from build123d import *
from build123d.topology import SkipClean

# Parameters (mm, degrees)
SZKIC1_W                   = 3.2
SZKIC1_H                   = 4.5
OBR_T1_ANGLE               = 180
OBR_T1_OTHER_WAY_ANGLE     = 180
WYTNIJ_WYCI_GNI_CIE1_DEPTH = 32.6


with BuildPart() as part:
    # Szkic1 → Obrót1 (revolve)
    with BuildSketch(Plane(origin=(0, 0, 0), x_dir=(1, 0, 0), z_dir=(0, 1, 0))):
        with Locations((1.6, 10.4)):
            Rectangle(SZKIC1_W, SZKIC1_H)
    revolve(axis=Axis((1, 0, 0), (-1, 0, 0)), revolution_arc=OBR_T1_ANGLE)

    # Szkic1 → Obrót1 other way (revolve)
    with SkipClean():  # the faces are left unmerged after this step: merging them gives an invalid solid
        with BuildSketch(Plane(origin=(0, 0, 0), x_dir=(1, 0, 0), z_dir=(0, 1, 0))):
            with Locations((1.6, 10.4)):
                Rectangle(SZKIC1_W, SZKIC1_H)
        revolve(axis=Axis((1, 0, 0), (1, 0, 0)), revolution_arc=OBR_T1_OTHER_WAY_ANGLE)

    # Szkic2 → Wytnij-wyciągnięcie1 (cut)
    with BuildSketch(Plane.XY):
        Polygon((-3.2, 0.302071906), (-3.2, -2.016946738), (4.85, 0.140044261), (4.85, 2.459062905), align=None)
    extrude(amount=WYTNIJ_WYCI_GNI_CIE1_DEPTH, mode=Mode.SUBTRACT)

    # Szkic3 → Wycięcie-obrót1 (revolve, cut)
    with BuildSketch(Plane.XY):
        with BuildLine():
            Line((0, 5.433333333), (3.2, 5.433333333))
            Line((3.2, 5.433333333), (3.2, 9.35))
            ThreePointArc((3.2, 9.35), (2.848528137, 8.501471863), (2, 8.15))
            Line((2, 8.15), (1.2, 8.15))
            ThreePointArc((1.2, 8.15), (0.351471863, 8.501471863), (0, 9.35))
            Line((0, 9.35), (0, 5.433333333))
        make_face()
    revolve(axis=Axis((1, 0, 0), (-1, 0, 0)), mode=Mode.SUBTRACT)


solid = part.part
Design review of the part built by this model. Coordinates are the model's own, in mm. Coordinates: 2 decimals unless noted, no trailing zeros. Loops run counter-clockwise (first coordinate to the right, second up) from the corner with the lowest first, then second, coordinate; pieces in that order, holes last. Notation, with made-up numbers: (51, -14.75) - (77, -14.75) arc R11 cw to (77, -4.75) - close; hole circle Ø5 at (66, 69). An arc over 180 degrees is marked (long way). Use CSV: the item, a comma, the result in double quotes. Start each with the question number.
1. Mouldability with a two-part tool opening along Y and no side actions: class faces 1 (the flat face through (1.622, 1.594, 10.25)), 2 (the flat face through (3.2, -6, -8)), 3 (the flat face through (1.578, -0.737, 10.344)) as released by +Y, released by -Y, zero draft, split by the parting line, or undercut.
2. Add section B-B on y = 10.25. Give the boundary of the cut face in (x, z).
3. To check wall thickness, follow probe 1 along Y at (x, z) = (1.65, 0); probe 2 along Y at (x, z) = (1.75, 3); probe 3 along Z at (x, y) = (1.85, -6.5). State the ranges of each line that lie inside material, in increasing order.
4. Clearance check with flat-ended pins moving along their axes: pin 1 (1.5 mm diameter, centred on x = 2, z = -5.5, fed in from -Y); pin 2 (10 mm diameter, centred on y = 0, z = 0, fed in from +X). State where each tip first meets the part, or that it passes through.
5. Add section C-C on z = -10. Give the boundary of the cut face in (x, y), plus the area to 3 significant figures.
6. Add section A-A on z = 0. Give the boundary of the cut face in (x, y).
Resolved:
1,face 1,"undercut"
1,face 2,"zero draft"
1,face 3,"undercut"
2,outline,"(0, -7.41) - (3.2, -7.41) - (3.2, 7.41) - (0, 7.41) - close"
3,probe 1,"-12.65 to -8.15, 8.15 to 12.65"
3,probe 2,"-12.29 to -7.58, 7.58 to 12.29"
3,probe 3,"-10.85 to -4.92, 4.92 to 10.85"
4,pin 1,"y = -11.72"
4,pin 2,"through"
5,outline,"(0, -7.75) - (3.2, -7.75) - (3.2, 7.75) - (0, 7.75) - close"
5,area,"49.6 mm2"
6,outline,"(0, -12.65) - (3.2, -12.65) - (3.2, -9.35) arc R1.2 ccw to (2, -8.15) - (1.2, -8.15) arc R1.2 ccw to (0, -9.35) - close; (0, 9.35) arc R1.2 ccw to (1.2, 8.15) - (2, 8.15) arc R1.2 ccw to (3.2, 9.35) - (3.2, 12.65) - (0, 12.65) - close"
